Read the model definition and answer for the solid it produces. Units are mm, in the model's axes. A direction names the side the tool comes from. Coordinates: 2 decimals unless noted, no trailing zeros. Loops run counter-clockwise (first coordinate to the right, second up) from the corner with the lowest first, then second, coordinate; pieces in that order, holes last. Notation, with made-up numbers: M 19.5,-22 L 28.5,-22 A15 ccw 28.5,-8 Z; hole C 15.5,11 d10. An arc over 180 degrees is marked long. Put each result on its own line as item: value.
from build123d import *

# Parameters (mm, degrees)
SKETCH2_W  = 5.5
SKETCH2_H  = 3
BODY_DEPTH = 3.75


with BuildPart() as part:
    # Sketch2 → Body (new, symmetric)
    with BuildSketch(Plane(origin=(0, 0, 0), x_dir=(1, 0, 0), z_dir=(0, 1, 0))):
        Polygon((-5, -6), (0, -26), (5, -6), (5, 0), (-5, 0), align=None)
        with Locations((0, -4.5)):
            Rectangle(SKETCH2_W, SKETCH2_H, mode=Mode.SUBTRACT)
    extrude(amount=BODY_DEPTH, both=True)


solid = part.part
1) Which of the six approach directions +Z, -Z, +X, -X, +Y, -Y give full straight-line access (tool end or side, diameter ignored) to faces 4 (the flat face through (-2.75, 0, 5)), 5 (the flat face through (0, -3.75, 10))?
Answer list:
face 4: +Y, -Y
face 5: +Z, -Z, +X, -X, -Y
2) Find section C-C, the plane x = 0.5. Write down the section's boundary in (y, z).
Answer list:
outline: M -3.75,0 L 3.75,0 L 3.75,3 L -3.75,3 Z; M -3.75,6 L 3.75,6 L 3.75,24 L -3.75,24 Z
3) Straight lines are drawn through the part: line 1 (X direction, y = -1, z = 4.5); line 2 (X direction, y = -1.5, z = 16); line 3 (X direction, y = -0.75, z = 16.5) (3 decimals). For each, find the intervals that lie inside material, in ascending order. Write a range as [from, to].
Answer list:
line 1: x = [-5, -2.75], [2.75, 5]
line 2: x = [-2.5, 2.5]
line 3: x = [-2.375, 2.375]
4) Determine the mould class of faces 1 (the flat face through (2.75, 0, 5)), 2 (the flat face through (-5, 0, 3)), 3 (the flat face through (2.465, 0.053, 16.14)) for opening direction X: released by +X, released by -X, zero draft, split by the parting line, or undercut.
Answer list:
face 1: undercut
face 2: released by -X
face 3: released by +X
5) Find section B-B, the plane y = 2. Write down the section's boundary in (x, z).
Answer list:
outline: M -5,0 L 5,0 L 5,6 L 0,26 L -5,6 Z; hole M -2.75,3 L 2.75,3 L 2.75,6 L -2.75,6 Z
6) Find section A-A, the plane x = -2.5. Write down the section's boundary in (y, z).
Answer list:
outline: M -3.75,0 L 3.75,0 L 3.75,3 L -3.75,3 Z; M -3.75,6 L 3.75,6 L 3.75,16 L -3.75,16 Z
7) Given pin 1 Ø2 at (y, z) = (1, 10) entering from +X; pin 2 Ø2 at (y, z) = (-2.5, 21.5) entering from +X (3 decimals); pin 3 Ø3 at (x, z) = (-3.5, 12.5) entering from +Y; pin 4 Ø1.5 at (y, z) = (1, 9.5) entering from +X, each flat-ended and moving along its own axis, determine where each tip first touches the part or whether it passes through.
Answer list:
pin 1: stops at x = 4.25
pin 2: stops at x = 1.375
pin 3: stops at y = 3.75
pin 4: stops at x = 4.31
8) Find section D-D, the plane z = 10. Write down the section's boundary in (x, y), plus the area to 3 significant figures.
Answer list:
outline: M -4,-3.75 L 4,-3.75 L 4,3.75 L -4,3.75 Z
area: 60.0 mm^2
